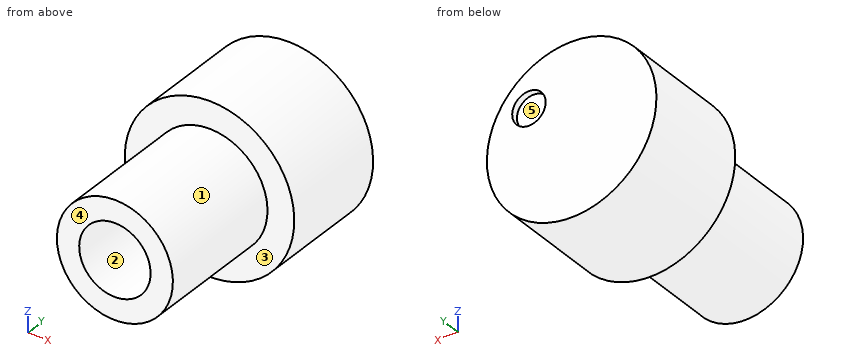
from build123d import *

# Parameters (mm, degrees)
SKETCH1_R           = 5.2
SKETCH1_R_2         = 3.2
BOSS_EXTRUDE1_DEPTH = 12
SKETCH2_R           = 7.6
BOSS_EXTRUDE2_DEPTH = 10
BOSS_EXTRUDE4_START = 5
BOSS_EXTRUDE4_DEPTH = 5
SKETCH5_R           = 1.5
CUT_EXTRUDE1_DEPTH  = 0.6


with BuildPart() as part:
    # Sketch1 → Boss-Extrude1 (new body)
    with BuildSketch(Plane(origin=(0, 0, 0), x_dir=(1, 0, 0), z_dir=(0, 1, 0))):
        with Locations(Location((0, 0, 0), (0, 0, 270))):
            Circle(SKETCH1_R)
        with Locations(Location((0, 0, 0), (0, 0, 270))):
            Circle(SKETCH1_R_2, mode=Mode.SUBTRACT)
    extrude(amount=BOSS_EXTRUDE1_DEPTH)

    # Sketch2 → Boss-Extrude2 (add)
    with BuildSketch(Plane(origin=(0, 12, 0), x_dir=(1, 0, 0), z_dir=(0, 1, 0))):
        with Locations(Location((0, 0, 0), (0, 0, 270))):
            Circle(SKETCH2_R)
    extrude(amount=BOSS_EXTRUDE2_DEPTH)

    # Sketch4 → Boss-Extrude4 (add)
    with BuildSketch(Plane.XZ.offset(-12).offset(BOSS_EXTRUDE4_START)):
        with BuildLine():
            Line((2.645751311, -1.8), (-2.645751311, -1.8))
            ThreePointArc((-2.645751311, -1.8), (0, -3.2), (2.645751311, -1.8))
        make_face()
    extrude(amount=-BOSS_EXTRUDE4_DEPTH)

    # Sketch5 → Cut-Extrude1 (cut)
    with BuildSketch(Plane(origin=(0, 22, 0), x_dir=(1, 0, 0), z_dir=(0, 1, 0))):
        with Locations(Location((3.830222216, -3.213938048, 0), (0, 0, 270))):
            Circle(SKETCH5_R)
    extrude(amount=-CUT_EXTRUDE1_DEPTH, mode=Mode.SUBTRACT)


solid = part.part
Here's how the part is built. I have some questions about the finished solid (model axes, mm). Face numbers are marked on the shaded views. A direction names the side the tool comes from. Give positions to 0.01 mm unless a question says otherwise; leave off trailing zeros. Order: outer loops, then holes, each group sorted by start corner. A loop starts at its lowest first (then second) coordinate and runs counter-clockwise, first axis right, second up. Notation, with made-up numbers: M -11.75,4.5 L 18.25,4.5 A18 ccw 18.25,25.5 Z; hole C 49.5,-27 d1. An arc over 180 degrees is marked long. Answer as a JSON object with one key per item and string values. Group by question number.
1) On a 3-axis mill with a long thin cutter (end or side, diameter ignored), from which of +Z, -Z, +X, -X, +Y, -Y can I reach the whole of each face in a straight line? I mean the marked faces 4 and 5. Say none if no direction works.
2) Suppose I cut it at A-A, the plane x = 0. Write out the boundary of the cut face in (y, z).
3) Please list where these lines run through material, in increasing order: L1, parallel to X at y = 7.25, z = 0; L2, parallel to Y at x = 0.25, z = -2.5; L3, parallel to Y at x = 4, z = -6.25. Write a range as [from, to].
4) Suppose I cut it at C-C, the plane z = 0. Write out the boundary of the cut face in (x, y).
5) Suppose I cut it at D-D, the plane y = 12.5. Write out the boundary of the cut face in (x, z).
6) We'd pull the mould along Z, two halves only. Please class the marked faces 1, 2 and 3: pulls with the +Z half, pulls with the -Z half, needs draft (parallel to the pull), parting line crosses it, or undercut.
7) Suppose I cut it at B-B, the plane y = 1.5. Write out the boundary of the cut face in (x, z).
8) I'm going to push flat-ended pins straight in: pin 1 Ø2 at (y, z) = (14, -5) entering from +X; pin 2 Ø1.5 at (x, y) = (0, 9) entering from -Z; pin 3 Ø2.5 at (x, y) = (-0.5, 9) entering from +Z. Where does each tip first touch, or does it pass through?
Results found:
{
 "1": {"face 4": "+Z, -Z, +X, -X, -Y", "face 5": "+Y"},
 "2": {"outline": "M 0,-5.2 L 12,-5.2 L 12,-7.6 L 22,-7.6 L 22,7.6 L 12,7.6 L 12,5.2 L 0,5.2 L 0,3.2 L 12,3.2 L 12,-1.8 L 7,-1.8 L 7,-3.2 L 0,-3.2 Z"},
 "3": {"L1": "[-5.2, -3.2], [3.2, 5.2]", "L2": "[7, 22]", "L3": "[12, 22]"},
 "4": {"outline": "M -7.6,12 L -5.2,12 L -5.2,0 L -3.2,0 L -3.2,12 L 3.2,12 L 3.2,0 L 5.2,0 L 5.2,12 L 7.6,12 L 7.6,22 L -7.6,22 Z"},
 "5": {"outline": "C 0,0 d15.2"},
 "6": {"face 1": "parting line crosses it", "face 2": "undercut", "face 3": "needs draft"},
 "7": {"outline": "C 0,0 d10.4; hole C 0,0 d6.4"},
 "8": {"pin 1": "x = 6.46", "pin 2": "z = -5.2", "pin 3": "z = 5.2"}
}
